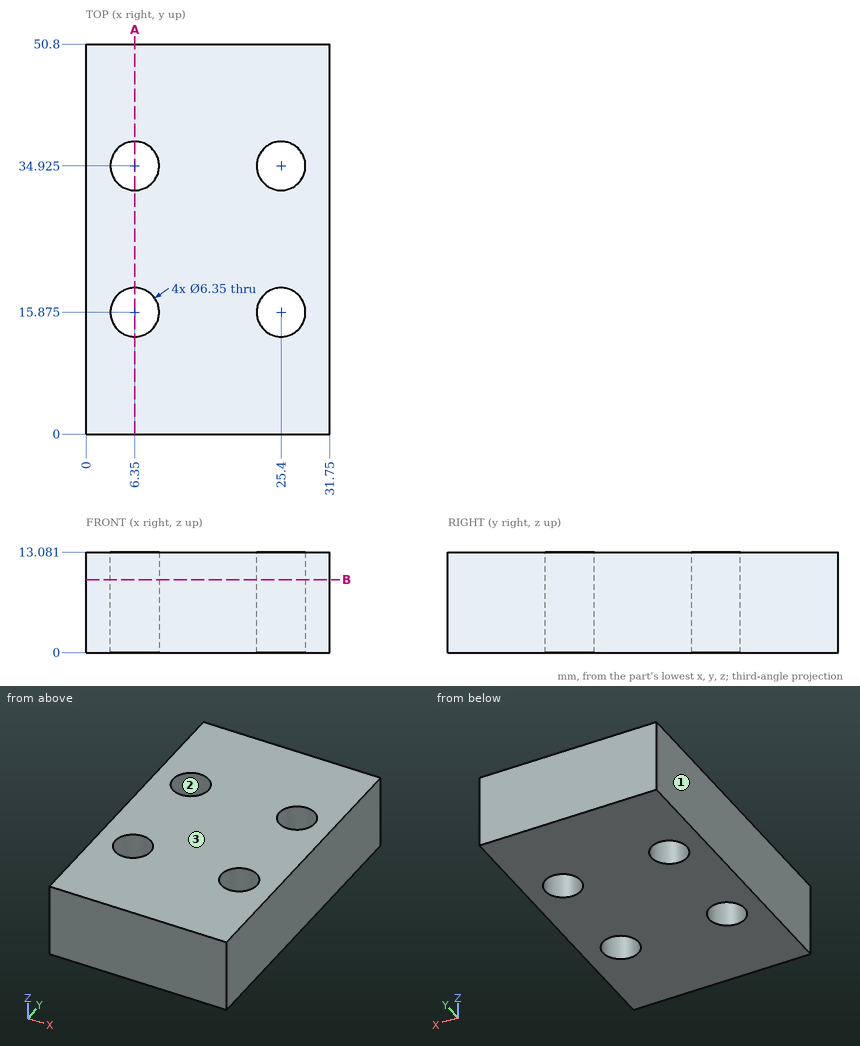
Here's the drawing with two shaded views (mm, measured from the low corner). I have some questions. Coordinates: 2 decimals unless noted, no trailing zeros. Loops run counter-clockwise (first coordinate to the right, second up) from the corner with the lowest first, then second, coordinate; pieces in that order, holes last. Notation, with made-up numbers: M 18,11.25 L 60,11.25 A17 cw 60,24.25 Z; hole C -4.75,84 d2. An arc over 180 degrees is marked long. Return JSON: item names as keys, results as strings. Group by question number.
Item 1: Imagine slicing it at B-B (z = 9.5). Please give me the cut outline in (x, y) (3 decimals).
Item 2: Thinking about a two-plate mould opening in X: for the marked faces 1, 2 and 3, which applies, released by +X, released by -X, zero draft, split by the parting line, or undercut?
Item 3: Imagine slicing it at A-A (x = 6.35). Please give me the cut outline in (y, z).
Item 4: If I drill on L1, parallel to Y at x = 25.4, z = 6.75; L2, parallel to Y at x = 4.5, z = 1; L3, parallel to X at y = 17.5, z = 3.5, over which ranges is the centre line in solid material (lowest first)? Write a range as from..to.
Item 5: I'm going to push a flat-ended pin straight in: pin 1 Ø12 at (x, y) = (6, 26) entering from -Z. Where does the tip first touch, or does it pass through?
Verdict:
{
 "1": {"outline": "M 0,0 L 31.75,0 L 31.75,50.8 L 0,50.8 Z; hole C 6.35,15.875 d6.35; hole C 6.35,34.925 d6.35; hole C 25.4,15.875 d6.35; hole C 25.4,34.925 d6.35"},
 "2": {"face 1": "released by -X", "face 2": "undercut", "face 3": "zero draft"},
 "3": {"outline": "M 0,0 L 12.7,0 L 12.7,13.08 L 0,13.08 Z; M 19.05,0 L 31.75,0 L 31.75,13.08 L 19.05,13.08 Z; M 38.1,0 L 50.8,0 L 50.8,13.08 L 38.1,13.08 Z"},
 "4": {"L1": "y = 0..12.7, 19.05..31.75, 38.1..50.8", "L2": "y = 0..13.29, 18.46..32.34, 37.51..50.8", "L3": "x = 0..3.62, 9.08..22.67, 28.13..31.75"},
 "5": {"pin 1": "stops at z = 0"}
}
